Geometry check sheet. Reference: the model listing, model coordinates, mm. A direction names the side the tool comes from. Give positions to 0.01 mm unless a question says otherwise; leave off trailing zeros. Loops run counter-clockwise (first coordinate to the right, second up) from the corner with the lowest first, then second, coordinate; pieces in that order, holes last.
1. Tool access check on faces 1 (the flat face through (17, 0, 1.65)), 2 (the flat face through (-18.968, -13, 1)). Record the directions out of +Z, -Z, +X, -X, +Y, -Y that give a thin tool (end or side, any length) a straight path to the whole face; none if there is none.
2. Cross-section at B-B, the plane z = -0.5. Record the cut outline in (x, y) (3 decimals), plus the area to 3 significant figures.
3. Cross-section at D-D, the plane y = -11.5. Record the cut outline in (x, z), plus the area to 3 significant figures.
4. Cross-section at A-A, the plane x = 0. Record the cut outline in (y, z) (3 decimals).
5. Release check for a two-part mould opening along Y. For faces 3 (the flat face through (-11.052, 18, 1)), 4 (the cylindrical face through (-36.574, 34.011, 0.306)), 5 (the flat face through (-17, 7.335, 1)), 6 (the flat face through (1, 8, -1)) record: +Y half, -Y half, draft (parallel to the pull), parting line (faces both ways), or undercut.
6. Material ranges on L1, parallel to Y at x = 15.5, z = 1.3 (3 decimals); L2, parallel to Y at x = 0, z = -0.5 (3 decimals); L3, parallel to X at y = -3.5, z = 0.95, recorded low to high.
7. Cross-section at C-C, the plane y = 0. Record the cut outline in (x, z), plus the area to 3 significant figures.
8. Go/stop test with flat-tipped pins: pin 1 Ø1 at (x, y) = (14.5, 9.5) entering from +Z; pin 2 Ø10 at (x, y) = (-16, -8.5) entering from +Z. Record where each tip stops, or that it passes through.
Solid Edge part; units mm, degrees
sketch "Sketch1" plane through (0, 0, 0) normal (0, 0, 1) x (1, 0, 0)
  line L0 (-15.01, -16.335) -> (-15.01, 16.335)
  line L1 (-15.01, 16.335) -> (15.01, 16.335)
  line L2 (15.01, 16.335) -> (15.01, -16.335)
  line L3 (15.01, -16.335) -> (-15.01, -16.335)
  line L4 (-38, -35.515) -> (-38, 35.515)
  line L5 (-38, 35.515) -> (38, 35.515)
  line L6 (38, 35.515) -> (38, -35.515)
  line L7 (38, -35.515) -> (-38, -35.515)
extrude "Protrusion1" add sketch "Sketch1" along normal blind 1.65
sketch "Sketch2" plane through (0, 0, 0) normal (0, 0, 1) x (1, 0, 0)
  line L0 (38, -35.515) -> (-38, -35.515)
  line L1 (-38, -35.515) -> (-38, 35.515)
  line L2 (-38, 35.515) -> (38, 35.515)
  line L3 (38, 35.515) -> (38, -35.515)
extrude "ExtrudedProtrusion_2" add sketch "Sketch2" against normal blind 1
sketch "Sketch3" plane through (0, 0, 1.65) normal (0, 0, 1) x (1, 0, 0)
  line L0 (-18.968, -7.185) -> (-4.68, -7.185)
  line L1 (-4.68, -7.185) -> (-4.68, -19.2068)
  line L2 (-4.68, -19.2068) -> (-18.968, -19.2068)
  line L3 (-18.968, -19.2068) -> (-18.968, -7.185)
  line L4 (-11.052, 7.335) -> (-11.052, 18.835)
  line L5 (-11.052, 18.835) -> (-18.968, 18.835)
  line L6 (-18.968, 18.835) -> (-18.968, 7.335)
  line L7 (-18.968, 7.335) -> (-11.052, 7.335)
  line L8 (-1.51, 13.835) -> (-6.51, 13.835)
  line L9 (-6.51, 13.835) -> (-6.51, 18.835)
  line L10 (-6.51, 18.835) -> (-1.51, 18.835)
  line L11 (-1.51, 18.835) -> (-1.51, 13.835)
  line L12 (11.8674, 7.335) -> (18.1526, 7.335)
  line L13 (18.1526, 7.335) -> (18.1526, 18.835)
  line L14 (18.1526, 18.835) -> (11.8674, 18.835)
  line L15 (11.8674, 18.835) -> (11.8674, 7.335)
  line L16 (9.1239, -19.2068) -> (9.1239, -7.185)
  line L17 (9.1239, -7.185) -> (18.1526, -7.185)
  line L18 (18.1526, -7.185) -> (18.1526, -19.2068)
  line L19 (18.1526, -19.2068) -> (9.1239, -19.2068)
extrude "Cutout1" cut sketch "Sketch3" against normal up to vertex (1.65 mm away)
fillet "Round_1" radius 0.7 5 edges at (-8.781, 16.335, 1.65) (5.1787, 16.335, 1.65) (15.01, 0.075, 1.65) (2.2219, -16.335, 1.65) (-15.01, 0.075, 1.65)
sketch "Sketch4" plane through (-0.4077, -0.1859, 0) normal (0, 0, 1) x (1, 0, 0)
  circle A0 centre (0.4077, 0.1859) radius 7.5
extrude "Cutout2" cut sketch "Sketch4" against normal up to next
fillet "Round_2" radius 5 4 edges at (38, -35.515, 0.325) (-38, -35.515, 0.325) (-38, 35.515, 0.325) (38, 35.515, 0.325)
Result:
1. face 1: +Z, +X, -X, +Y, -Y
1. face 2: +Z
2. outline: (-38, -30.515) arc R5 ccw to (-33, -35.515) - (33, -35.515) arc R5 ccw to (38, -30.515) - (38, 30.515) arc R5 ccw to (33, 35.515) - (-33, 35.515) arc R5 ccw to (-38, 30.515) - close; hole circle Ø15 at (0, 0)
2. area: 5,200 mm2
3. outline: (-38, -1) - (38, -1) - (38, 1.65) - (18.15, 1.65) - (18.15, 0) - (-18.97, 0) - (-18.97, 1.65) - (-38, 1.65) - close
3. area: 140 mm2
4. outline: (-35.515, -1) - (-7.5, -1) - (-7.5, 0) - (-16.335, 0) - (-16.335, 0.95) arc R0.7 ccw to (-17.035, 1.65) - (-35.515, 1.65) - close; (7.5, -1) - (35.515, -1) - (35.515, 1.65) - (17.035, 1.65) arc R0.7 ccw to (16.335, 0.95) - (16.335, 0) - (7.5, 0) - close
5. face 3: undercut
5. face 4: +Y half
5. face 5: undercut
5. face 6: draft
6. L1: y = -35.515 to -19.207, -7.185 to 7.335, 18.835 to 35.515
6. L2: y = -35.515 to -7.5, 7.5 to 35.515
6. L3: x = -38 to -15.01, 15.01 to 38
7. outline: (-38, -1) - (-7.5, -1) - (-7.5, 0) - (-15.01, 0) - (-15.01, 0.95) arc R0.7 ccw to (-15.71, 1.65) - (-38, 1.65) - close; (7.5, -1) - (38, -1) - (38, 1.65) - (15.71, 1.65) arc R0.7 ccw to (15.01, 0.95) - (15.01, 0) - (7.5, 0) - close
7. area: 137 mm2
8. pin 1: stops at z = 0
8. pin 2: stops at z = 1.65
